Read the model definition and answer for the solid it produces. Units are mm, in the model's axes. A direction names the side the tool comes from. Coordinates: 2 decimals unless noted, no trailing zeros. Loops run counter-clockwise (first coordinate to the right, second up) from the corner with the lowest first, then second, coordinate; pieces in that order, holes last. Notation, with made-up numbers: (8.5, -26) - (39.5, -26) arc R28 ccw to (39.5, 3) - close; hole circle Ø7 at (-36.5, 82.25). An arc over 180 degrees is marked (long way). Use one line per item in the form item = value. Start each with the question number.
1) A cutting plane is placed at C-C (y = -24.13). Give the vertices of the cut face in (x, z), and give its area (3 significant figures).
2) A cutting plane is placed at D-D (x = 23). Give the vertices of the cut face in (y, z), and give its area (3 significant figures).
3) Each of these flat-tipped pins is pushed along its axis until it touches: P1, Ø20.5, axis at y = 0, z = 0, coming from the -X side; P2, Ø5, axis at x = 6.5, y = -20.5, coming from the +Z side; P3, Ø16, axis at y = 24.13, z = 0, coming from the +X side; P4, Ø1, axis at y = -9, z = 30.5, coming from the +X side. Where does it stop, or does it pass through?
4) Which of the six approach directions +Z, -Z, +X, -X, +Y, -Y give full straight-line access (tool end or side, diameter ignored) to faces 1 (the face through (10.16, -31, -20)), 2 (the face through (13, 7.938, 0)), 3 (the face through (0, -8, -1))?
5) The mould has two halves that part along Y. Classify faces 4 (the face through (6.439, 17.474, -27.952)), 5 (the face through (25.4, 6, -3)), 6 (the face through (1.252, -38.806, -8.617)), 7 (the face through (13, 7, 1.588)): released by +Y, released by -Y, zero draft, split by the parting line, or undercut.
6) A cutting plane is placed at A-A (z = 0). Give the vertices of the cut face in (x, y), and give its area (3 significant figures).
7) Consider line 1 (Y direction, x = 3.25, z = 0); line 2 (Y direction, x = 6.5, z = 24); line 3 (Y direction, x = 21.5, z = 0). Determine where each line is inside the solid, lowest interval first.
8) A cutting plane is placed at B-B (y = -9). Give the vertices of the cut face in (x, z), and give its area (3 significant figures).
from build123d import *

# Parameters (mm, degrees)
SKETCH1_R           = 25.4
BOSS_EXTRUDE1_DEPTH = 25.4
SKETCH2_R           = 38.1
SKETCH2_R_2         = 10.9140625
BOSS_EXTRUDE2_DEPTH = 12.7
SKETCH3_R           = 25.4
SKETCH3_R_2         = 12.7
CUT_EXTRUDE1_DEPTH  = 12.7
SKETCH4_R           = 8.89
CUT_EXTRUDE2_DEPTH  = 13.7
CIRPATTERN1_COUNT   = 6
SKETCH5_R           = 39.751
SKETCH5_R_2         = 38.1
BOSS_EXTRUDE3_DEPTH = 2.54
SKETCH6_R           = 38.1
SKETCH6_R_2         = 36.449
CUT_EXTRUDE3_DEPTH  = 2.54


with BuildPart() as part:
    # Sketch1 → Boss-Extrude1 (new body)
    with BuildSketch(Plane(origin=(0, 0, 0), x_dir=(0, 0, -1), z_dir=(1, 0, 0))):
        Circle(SKETCH1_R)
        with BuildLine():
            Line((-1.5875, 6.148361062), (-1.5875, 7.9375))
            Line((-1.5875, 7.9375), (1.5875, 7.9375))
            Line((1.5875, 7.9375), (1.5875, 6.148361062))
            ThreePointArc((1.5875, 6.148361062), (5.020115786, 3.888564967), (6.35, 0))
            ThreePointArc((6.35, 0), (-3.888564967, -5.020115786), (-1.5875, 6.148361062))
        make_face(mode=Mode.SUBTRACT)
    extrude(amount=BOSS_EXTRUDE1_DEPTH)

    # Sketch2 → Boss-Extrude2 (add)
    with BuildSketch(Plane.ZY):
        Circle(SKETCH2_R)
        Circle(SKETCH2_R_2, mode=Mode.SUBTRACT)
    extrude(amount=-BOSS_EXTRUDE2_DEPTH)

    # Sketch3 → Cut-Extrude1 (cut)
    with BuildSketch(Plane(origin=(25.4, 0, 0), x_dir=(0, 0, -1), z_dir=(1, 0, 0))):
        Circle(SKETCH3_R)
        Circle(SKETCH3_R_2, mode=Mode.SUBTRACT)
    extrude(amount=-CUT_EXTRUDE1_DEPTH, mode=Mode.SUBTRACT)

    # Sketch4 → Cut-Extrude2 (cut, through all)
    with BuildSketch(Plane(origin=(12.7, 0, 0), x_dir=(0, 0, -1), z_dir=(1, 0, 0))):
        with Locations((0, 24.13)):
            Circle(SKETCH4_R)
    cut_extrude2 = extrude(amount=-CUT_EXTRUDE2_DEPTH, mode=Mode.SUBTRACT)

    # CirPattern1: Cut-Extrude2 ×6 about axis
    cirpattern1_axis = Axis((0, 0, 0), (1, 0, 0))
    for i in range(1, CIRPATTERN1_COUNT):
        add(cut_extrude2.rotate(cirpattern1_axis, i * 360 / CIRPATTERN1_COUNT), mode=Mode.SUBTRACT)

    # Sketch5 → Boss-Extrude3 (add)
    with BuildSketch(Plane.ZY):
        Circle(SKETCH5_R)
        Circle(SKETCH5_R_2, mode=Mode.SUBTRACT)
    extrude(amount=-BOSS_EXTRUDE3_DEPTH)

    # Sketch6 → Cut-Extrude3 (cut)
    with BuildSketch(Plane(origin=(12.7, 0, 0), x_dir=(0, 0, -1), z_dir=(1, 0, 0))):
        Circle(SKETCH6_R)
        Circle(SKETCH6_R_2, mode=Mode.SUBTRACT)
    extrude(amount=-CUT_EXTRUDE3_DEPTH, mode=Mode.SUBTRACT)


solid = part.part
Found:
q1.outline = (0, -31.59) - (2.54, -31.59) - (2.54, -29.48) - (10.16, -29.48) - (10.16, -27.32) - (12.7, -27.32) - (12.7, -8.89) - (0, -8.89) - close; (0, 8.89) - (12.7, 8.89) - (12.7, 27.32) - (10.16, 27.32) - (10.16, 29.48) - (2.54, 29.48) - (2.54, 31.59) - (0, 31.59) - close
q1.area = 523 mm^2
q2.outline = circle Ø25.4 at (0, 0); hole (6.15, -1.59) - (7.94, -1.59) - (7.94, 1.59) - (6.15, 1.59) arc R6.35 ccw (long way) to start
q2.area = 375 mm^2
q3.P1 = 0
q3.P2 = 33.58
q3.P3 = through
q3.P4 = 12.7
q4.face_1 = +X
q4.face_2 = +X, -X
q4.face_3 = +Z, -Z, -X, +Y, -Y
q5.face_4 = undercut
q5.face_5 = zero draft
q5.face_6 = split by the parting line
q5.face_7 = undercut
q6.outline = (0, -39.75) - (2.54, -39.75) - (2.54, -38.1) - (10.16, -38.1) - (10.16, -36.45) - (12.7, -36.45) - (12.7, -33.02) - (0, -33.02) - close; (0, -15.24) - (12.7, -15.24) - (12.7, -12.7) - (25.4, -12.7) - (25.4, -6.35) - (0, -6.35) - close; (0, 7.94) - (25.4, 7.94) - (25.4, 12.7) - (12.7, 12.7) - (12.7, 15.24) - (0, 15.24) - close; (0, 33.02) - (12.7, 33.02) - (12.7, 36.45) - (10.16, 36.45) - (10.16, 38.1) - (2.54, 38.1) - (2.54, 39.75) - (0, 39.75) - close
q6.area = 476 mm^2
q7.line_1 = -38.1 to -33.02, -15.24 to -6.35, 7.94 to 15.24, 33.02 to 38.1
q7.line_2 = -29.59 to -20.4, -3.73 to 3.73, 20.4 to 29.59
q7.line_3 = -12.7 to -6.35, 7.94 to 12.7
q8.outline = (0, -38.72) - (2.54, -38.72) - (2.54, -37.02) - (10.16, -37.02) - (10.16, -35.32) - (12.7, -35.32) - (12.7, -29.24) - (0, -29.24) - close; (0, -12.55) - (12.7, -12.55) - (12.7, -8.96) - (25.4, -8.96) - (25.4, 8.96) - (12.7, 8.96) - (12.7, 12.55) - (0, 12.55) - close; (0, 29.24) - (12.7, 29.24) - (12.7, 35.32) - (10.16, 35.32) - (10.16, 37.02) - (2.54, 37.02) - (2.54, 38.72) - (0, 38.72) - close
q8.area = 744 mm^2
